Can you work these out from the model? Positions are in its coordinate system, mm. Face numbers are marked on the shaded views. Round coordinates to 2 decimals unless told otherwise and drop trailing zeros. Order: outer loops, then holes, each group sorted by start corner. A loop starts at its lowest first (then second) coordinate and runs counter-clockwise, first axis right, second up. Notation, with made-up numbers: M -13.5,46.5 L 25.5,46.5 A8 cw 25.5,61.5 Z; hole C -18.5,78.25 d2. An arc over 180 degrees is marked long. Answer as a JSON object with one key per item and string values. Group by question number.
```python
from build123d import *

# Parameters (mm, degrees)
F0_W     = 22
F0_H     = 15
F1_DEPTH = 1.5
F2_W     = 22
F2_H     = 15
F2_W_2   = 19
F2_H_2   = 12
F3_DEPTH = 18
F4_SIZE  = 0.5
F5_SIZE  = 1


with BuildPart() as f1:
    # F0 (on Top) → F1 (new body)
    with BuildSketch(Plane.XY):
        with Locations((11, 7.5)):
            Rectangle(F0_W, F0_H)
    extrude(amount=F1_DEPTH)

    # F2 (on face) → F3 (join)
    with BuildSketch(Plane.XY.offset(1.5)):
        with Locations((11, 7.5)):
            Rectangle(F2_W, F2_H)
        with Locations((11, 7.5)):
            Rectangle(F2_W_2, F2_H_2, mode=Mode.SUBTRACT)
    extrude(amount=F3_DEPTH)

    # F4
    f4_edges = [f1.edges().sort_by_distance(p)[0] for p in [
        (0, 7.5, 0),
        (11, 0, 0),
        (22, 7.5, 0),
        (11, 15, 0),
        (22, 0, 9.75),
        (22, 15, 9.75),
        (0, 0, 9.75),
        (0, 15, 9.75),
    ]]
    chamfer(f4_edges, length=F4_SIZE)

    # F5
    f5_edges = [f1.edges().sort_by_distance(p)[0] for p in [
        (1.5, 7.5, 1.5),
        (11, 13.5, 1.5),
        (20.5, 7.5, 1.5),
        (11, 1.5, 1.5),
        (20.5, 13.5, 10.5),
        (1.5, 13.5, 10.5),
        (1.5, 1.5, 10.5),
        (20.5, 1.5, 10.5),
    ]]
    chamfer(f5_edges, length=F5_SIZE)


solid = f1.part
```
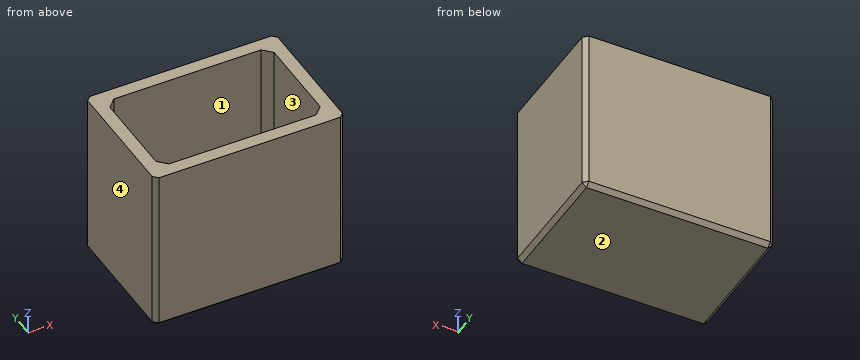
1) For pin 1 (6 mm diameter, centred on x = 14, y = 6, fed in from +Z), with a flat end and sliding along its axis, tell me the tip position at first contact or that it passes through.
2) I need wall thicknesses on line 1 along X through (y, z) = (4.25, 7.5); line 2 along Y through (x, z) = (13.25, 18); line 3 along Z through (x, y) = (6, 7). Which ranges of each line are inside material? Lowest first, please.
3) If we section it at A-A on z = 11: Write out the boundary of the cut face in (x, y), plus the area to 4 significant figures.
4) We'd pull the mould along X, two halves only. Please class the marked faces 1, 2, 3 and 4: +X half, -X half, draft (parallel to the pull), parting line (faces both ways), or undercut.
5) If we section it at B-B on y = 8: Write out the boundary of the cut face in (x, z), plus the area to 4 significant figures.
6) If we section it at C-C on x = 5.5: Write out the boundary of the cut face in (y, z).
Findings:
{
 "1": {"pin 1": "stops at z = 1.5"},
 "2": {"line 1": "x = 0 to 1.5, 20.5 to 22", "line 2": "y = 0 to 1.5, 13.5 to 15", "line 3": "z = 0 to 1.5"},
 "3": {"outline": "M 0,0.5 L 0.5,0 L 21.5,0 L 22,0.5 L 22,14.5 L 21.5,15 L 0.5,15 L 0,14.5 Z; hole M 1.5,2.5 L 2.5,1.5 L 19.5,1.5 L 20.5,2.5 L 20.5,12.5 L 19.5,13.5 L 2.5,13.5 L 1.5,12.5 Z", "area": "103.5 mm^2"},
 "4": {"face 1": "undercut", "face 2": "draft", "face 3": "undercut", "face 4": "-X half"},
 "5": {"outline": "M 0,0.5 L 0.5,0 L 21.5,0 L 22,0.5 L 22,19.5 L 20.5,19.5 L 20.5,2.5 L 19.5,1.5 L 2.5,1.5 L 1.5,2.5 L 1.5,19.5 L 0,19.5 Z", "area": "87.75 mm^2"},
 "6": {"outline": "M 0,0.5 L 0.5,0 L 14.5,0 L 15,0.5 L 15,19.5 L 13.5,19.5 L 13.5,2.5 L 12.5,1.5 L 2.5,1.5 L 1.5,2.5 L 1.5,19.5 L 0,19.5 Z"}
}
